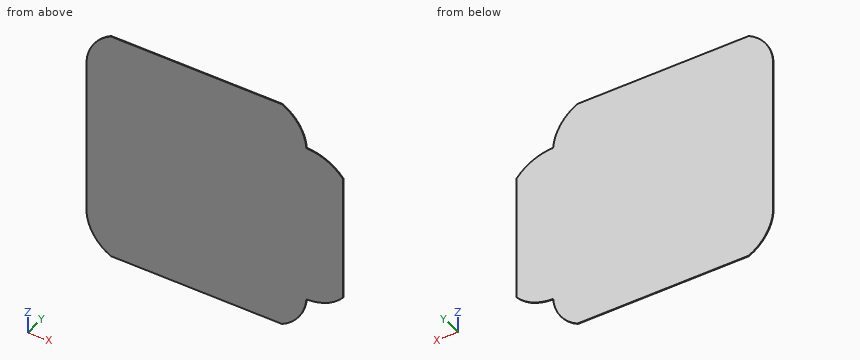
```python
from build123d import *

# Parameters (mm, degrees)
F0_W     = 300
F0_H     = 220
F1_DEPTH = 1


with BuildPart() as f1:
    # F0 (on Front) → F1 (new body)
    with BuildSketch(Plane.XZ):
        with BuildLine():
            Line((85.809135, 104.238631), (-147.819877, 104.238631))
            ThreePointArc((-147.819877, 104.238631), (-171.001324, 83.611616), (-181.005371, 54.238631))
            Line((-181.005371, 54.238631), (118.994629, 54.238631))
            ThreePointArc((118.994629, 54.238631), (108.990582, 83.611616), (85.809135, 104.238631))
        make_face()
        with Locations((-31.005371, -55.761369)):
            Rectangle(F0_W, F0_H)
        with BuildLine():
            ThreePointArc((168.994629, 30.675642), (146.5507, 47.881048), (118.994629, 54.238631))
            Line((118.994629, 54.238631), (118.994629, -165.761369))
            ThreePointArc((118.994629, -165.761369), (146.5507, -159.403787), (168.994629, -142.198381))
            Line((168.994629, -142.198381), (168.994629, 30.675642))
        make_face()
        with BuildLine():
            Line((118.994629, -165.761369), (-181.005371, -165.761369))
            ThreePointArc((-181.005371, -165.761369), (-171.001324, -195.134355), (-147.819877, -215.761369))
            Line((-147.819877, -215.761369), (85.809135, -215.761369))
            ThreePointArc((85.809135, -215.761369), (108.990582, -195.134355), (118.994629, -165.761369))
        make_face()
    extrude(amount=F1_DEPTH)


solid = f1.part
```
The listing builds one solid part. Answer for the finished solid, in the listing's coordinates (mm). Coordinates: 2 decimals unless noted, no trailing zeros. Loops run counter-clockwise (first coordinate to the right, second up) from the corner with the lowest first, then second, coordinate; pieces in that order, holes last. Notation, with made-up numbers: (41.5, 10) - (48.5, 10) arc R21 cw to (48.5, 15) - close; hole circle Ø2 at (-19.75, -27). An arc over 180 degrees is marked (long way). Write item = value, one per line.
1) Section B-B (z = -183.5) is taken. Determine the outline of the cut face in (x, y).
Responses:
outline = (-177.03, -1) - (115.02, -1) - (115.02, 0) - (-177.03, 0) - close
2) Section A-A (y = -0.6) is taken. Determine the outline of the cut face in (x, z), plus the area to 3 significant figures.
Responses:
outline = (-181.01, -165.76) arc R60.88 ccw to (-147.82, -215.76) - (85.81, -215.76) arc R60.88 ccw to (118.99, -165.76) arc R66.69 ccw to (168.99, -142.2) - (168.99, 30.68) arc R66.69 ccw to (118.99, 54.24) arc R60.88 ccw to (85.81, 104.24) - (-147.82, 104.24) arc R60.88 ccw to (-181.01, 54.24) - close
area = 104,000 mm^2
3) Section C-C (z = 67) is taken. Determine the outline of the cut face in (x, y).
Responses:
outline = (-178.72, -1) - (116.71, -1) - (116.71, 0) - (-178.72, 0) - close
4) Find the intervals of material crossed by line 1 along X through (y, z) = (-0.55, -183); line 2 along X through (y, z) = (-0.9, 67); line 3 along Z through (x, y) = (106, -0.35), in increasing order.
Responses:
line_1 = -177.22 to 115.21
line_2 = -178.72 to 116.71
line_3 = -199.26 to 87.73
